```python
from build123d import *

# Parameters (mm, degrees)
BOSS_EXTRUDE1_DEPTH = 300
FILLET1_R           = 5
SKETCH2_R           = 1
CUT_EXTRUDE3_DEPTH  = 2


# Read off the part's stored shape, not the designer's step: Boss-Extrude1
with BuildPart() as part:
    # Boss-Extrude1 outline → Boss-Extrude1 (new body)
    with BuildSketch(Plane.YZ):
        Polygon((0, -70), (10.675473791, -70), (3.318177323, 0), (0, 0), align=None)
    extrude(amount=BOSS_EXTRUDE1_DEPTH)

    # Fillet1
    fillet1_edges = [part.edges().sort_by_distance(p)[0] for p in [
        (300, 5.337736895, -70),
        (300, 1.659088662, 0),
        (0, 1.659088662, 0),
        (0, 5.337736895, -70),
    ]]
    fillet(fillet1_edges, radius=FILLET1_R)

    # Sketch2 → Cut-Extrude3 (cut)
    with BuildSketch(Plane.XZ):
        with BuildLine():
            ThreePointArc((151, -39), (152, -40), (153, -39))
            Line((153, -39), (153, -25))
            ThreePointArc((153, -25), (152, -24), (151, -25))
            Line((151, -25), (151, -34))
            Line((151, -34), (149, -34))
            ThreePointArc((149, -34), (148, -35), (149, -36))
            Line((149, -36), (151, -36))
            Line((151, -36), (151, -39))
        make_face()
        with BuildLine():
            Line((157.5, -31.5), (157.5, -21))
            ThreePointArc((157.5, -21), (156.5, -20), (155.5, -21))
            Line((155.5, -21), (155.5, -31.5))
            ThreePointArc((155.5, -31.5), (156.5, -32.5), (157.5, -31.5))
        make_face()
        with BuildLine():
            Line((148.2, -31.5), (148.2, -25.5))
            ThreePointArc((148.2, -25.5), (147.2, -24.5), (146.2, -25.5))
            Line((146.2, -25.5), (146.2, -31.5))
            ThreePointArc((146.2, -31.5), (147.2, -32.5), (148.2, -31.5))
        make_face()
        with BuildLine():
            Line((144.7, -31.5), (144.7, -25.5))
            ThreePointArc((144.7, -25.5), (143.7, -24.5), (142.7, -25.5))
            Line((142.7, -25.5), (142.7, -31.5))
            ThreePointArc((142.7, -31.5), (143.7, -32.5), (144.7, -31.5))
        make_face()
        with BuildLine():
            Line((141.2, -31.5), (141.2, -25.5))
            ThreePointArc((141.2, -25.5), (140.2, -24.5), (139.2, -25.5))
            Line((139.2, -25.5), (139.2, -31.5))
            ThreePointArc((139.2, -31.5), (140.2, -32.5), (141.2, -31.5))
        make_face()
        with BuildLine():
            Line((161, -23.5), (161, -21))
            ThreePointArc((161, -21), (160, -20), (159, -21))
            Line((159, -21), (159, -23.5))
            ThreePointArc((159, -23.5), (160, -24.5), (161, -23.5))
        make_face()
        with Locations(Location((156.5, -35, 0), (0, 0, 270))):
            Circle(SKETCH2_R)
    extrude(amount=-CUT_EXTRUDE3_DEPTH, mode=Mode.SUBTRACT)


solid = part.part
```
Design review of the part built by this model. Coordinates are the model's own, in mm. Give positions to 0.01 mm unless a question says otherwise; leave off trailing zeros. Order: outer loops, then holes, each group sorted by start corner. A loop starts at its lowest first (then second) coordinate and runs counter-clockwise, first axis right, second up. Notation, with made-up numbers: (22, 30.5) - (44, 30.5) arc R12 cw to (44, 44.5) - close; hole circle Ø4 at (-13.5, 66.25). An arc over 180 degrees is marked (long way). Use a Markdown table: item, result. Add a question column.
(1) Mouldability with a two-part tool opening along Z and no side actions: class faces 1 (the face through (300, 4, -41)), 2 (the face through (152, 2, -32)), 3 (the face through (148, 5, -70)) as +Z half, -Z half, draft (parallel to the pull), parting line (faces both ways), or undercut.
(2) Add section A-A on y = 7.5. Give the boundary of the cut face in (x, z).
(3) Wall thickness on probe 1 along Z at (x, y) = (156.5, 1.1); probe 2 along X at (y, z) = (0.6, -35); probe 3 along X at (y, z) = (1.25, -33.5): over which ranges is each line inside the solid? List them lowest first. Write a range as [from, to].
(4) Clearance check with a flat-ended pin moving along its axis: P1, Ø0.6, axis at x = 140, z = -28.5, coming from the -Y side. State where the tip first meets the part, or that it passes through.
(5) Add section B-B on x = 105.5. Give the boundary of the cut face in (y, z).
(6) Add section C-C on z = -16. Give the boundary of the cut face in (x, y), then the cut area to 3 significant figures.
Report:
| question | item | result |
|---|---|---|
| 1 | face 1 | draft |
| 1 | face 2 | undercut |
| 1 | face 3 | -Z half |
| 2 | outline | (0, -65) arc R5 ccw to (5, -70) - (295, -70) arc R5 ccw to (300, -65) - (300, -39.79) - (0, -39.79) - close |
| 3 | probe 1 | z = [-70, -36], [-34, -32.5], [-20, 0] |
| 3 | probe 2 | x = [0, 148], [153, 155.5], [157.5, 300] |
| 3 | probe 3 | x = [0, 151], [153, 300] |
| 4 | P1 | stops at y = 2 |
| 5 | outline | (0, -70) - (10.68, -70) - (3.32, 0) - (0, 0) - close |
| 6 | outline | (0, 0) - (300, 0) - (300, 5) - (0, 5) - close |
| 6 | area | 1,500 mm² |
